Read the model definition and answer for the solid it produces. Units are mm, in the model's axes. A direction names the side the tool comes from. Coordinates: 2 decimals unless noted, no trailing zeros. Loops run counter-clockwise (first coordinate to the right, second up) from the corner with the lowest first, then second, coordinate; pieces in that order, holes last. Notation, with made-up numbers: M -33,68.5 L -7,68.5 A25 ccw -7,94.5 Z; hole C 87,58.5 d9. An arc over 180 degrees is marked long. One line per item, written item: value. Start each with the question number.
Autodesk Fusion 360 part; units mm, degrees
sketch "Sketch1" plane through (0, 0, 0) normal (0, 1, 0) x (1, 0, 0)
  circle A0 centre (0, 0) radius 20
  circle A1 centre (0, 0) radius 21.5
  dimension "d1" = 40
  dimension "d2" = 1.5
extrude "Extrude1" add sketch "Sketch1" along normal blind 100

Autodesk Fusion 360 part; units mm, degrees
sketch "Sketch1" plane through (0, 0, 0) normal (0, 1, 0) x (1, 0, 0)
  circle A0 centre (0, 0) radius 18.5
  circle A1 centre (0, 0) radius 20
  dimension "d1" = 37
  dimension "d2" = 1.5
extrude "Extrude1" add sketch "Sketch1" along normal blind 15 draft 5 and the other way blind 5
sketch "Sketch2" plane through (0, 15, 0) normal (0, 1, 0) x (-1, 0, 0)
  circle A0 centre (0, 0) radius 17.1877
  circle A1 centre (0, 0) radius 21.3123
  circle A2 centre (0, 0) radius 17.1877
  circle A3 centre (0, 0) radius 21.3123
extrude "Extrude2" add sketch "Sketch2" along normal blind 10 draft 45
sketch "Sketch3" plane through (0, 25, 0) normal (0, 1, 0) x (-1, 0, 0)
  circle A0 centre (0, 0) radius 7.1877
  circle A1 centre (0, 0) radius 31.3123
  circle A2 centre (0, 0) radius 12.1877
  circle A3 centre (0, 0) radius 26.3123
extrude "Extrude3" add sketch "Sketch3" along normal blind 10 draft 50 contours A1 | A3
sketch "Sketch4" plane through (0, 25, 0) normal (0, 1, 0) x (-1, 0, 0)
  circle A0 centre (0, 0) radius 12.1877
  circle A1 centre (0, 0) radius 7.1877
  circle A2 centre (0, 0) radius 7.1877
extrude "Extrude4" cut sketch "Sketch4" along normal blind 60 contours A1 A2
sketch "Sketch5" plane through (0, 35, 0) normal (0, 1, 0) x (-1, 0, 0)
  circle A0 centre (0, 0) radius 7.1877
  circle A1 centre (0, 0) radius 43.2299
  circle A2 centre (0, 0) radius 35
extrude "Extrude5" cut sketch "Sketch5" against normal blind 20 draft -50 contours A2
ref_plane "WorkPlane1" through (0, 15, 0) normal (0, 1, 0) x (0, 0, 1)
sketch "Sketch6" plane through (0, 15, 0) normal (0, 1, 0) x (1, 0, 0)
  circle A0 centre (0, 0) radius 19
  dimension "d16" = 38
extrude "Extrude6" cut sketch "Sketch6" along normal blind -70 and the other way blind -65
sketch "Sketch7" plane through (0, 15, 0) normal (0, 1, 0) x (1, 0, 0)
  circle A0 centre (0, 0) radius 19
extrude "Extrude7" add sketch "Sketch7" against normal blind 15
sketch "Sketch8" plane through (0, 0, 0) normal (0, -1, 0) x (1, 0, 0)
  circle A0 centre (0, 0) radius 19
  circle A1 centre (0, 0) radius 19
extrude "Extrude8" add sketch "Sketch8" along normal blind 10 draft -60
sketch "Sketch9" plane through (0, -10, 0) normal (0, -1, 0) x (1, 0, 0)
  circle A0 centre (0, 0) radius 1.6795
  circle A1 centre (0, 0) radius 1.6795
  dimension "d27" = 3.359
extrude "Extrude9" cut sketch "Sketch9" against normal blind 60
1) A tool of negligible diameter and unlimited length cuts with its end or side. For faces 1 (the face through (4.1, 80, 18.2)), 2 (the face through (18, -5, 7)), 3 (the face through (-4.01, 89.86, -18.06)), from which of +Z, -Z, +X, -X, +Y, -Y can it reach the whole face along a straight path? Write none if from no direction.
2) Section D-D (y = 4) is taken. Determine the outline of the cut face in (x, z).
3) Flat-ended cylindrical pins translate along their axes: pin 1 (1 mm diameter, centred on x = 30.5, z = 13, fed in from -Y); pin 2 (12 mm diameter, centred on x = -4, y = 20.5, fed in from +Z); pin 3 (6 mm diameter, centred on x = 11, z = -27.5, fed in from +Y). Find the tip coordinate at first contact, or state that the pin passes through.
4) Consider line 1 along Z through (x, y) = (0, 92); line 2 along Z through (x, y) = (0, 41.5). Determine where each line is inside the solid, lowest interval first.
5) Section B-B (y = 74.5) is taken. Determine the outline of the cut face in (x, z), then the cut area to 3 significant figures.
6) For a pull along Z with two mould halves and no side action, classify faces 4 (the face through (8.767, 47.955, 16.856)), 5 (the face through (-19, 35, -9)), 6 (the face through (-4.336, -2.465, 19.524)) as released by +Z, released by -Z, zero draft, split by the parting line, or undercut.
Results found:
1. face 1: none
1. face 2: -Y
1. face 3: +Y
2. outline: C 0,0 d40.7; hole C 0,0 d3.36
3. pin 1: stops at y = 26.13
3. pin 2: stops at z = 32.89
3. pin 3: stops at y = 35
4. line 1: z = -20 to -18.5, 18.5 to 20
4. line 2: z = -20 to -19, 19 to 20
5. outline: C 0,0 d40; hole C 0,0 d38
5. area: 123 mm²
6. face 4: undercut
6. face 5: zero draft
6. face 6: split by the parting line
